from build123d import *

# Parameters (mm, degrees)
BOSS_EXTRUDE1_DEPTH                = 40.005
F_4_40_FOR_NUT_VERTICAL_DEPTH      = 82.258355524
F_4_40_FOR_NUT_VERTICAL_DEPTH_BACK = 82.258355524
SKETCH3_R                          = 1.4732
SKETCH3_R_2                        = 7.9375
SKETCH4_R                          = 3.2639
F_1_4_20_MOUNTING_DEPTH            = 82.258355524


with BuildPart() as part:
    # Sketch2 → Boss-Extrude1 (new body)
    with BuildSketch(Plane.XY):
        with BuildLine():
            Line((0, 5.842), (0, 50.0126))
            Line((0, 50.0126), (2.9972, 50.0126))
            Line((2.9972, 50.0126), (2.9972, 6.1722))
            ThreePointArc((2.9972, 6.1722), (3.92713597, 3.92713597), (6.1722, 2.9972))
            Line((6.1722, 2.9972), (50.0126, 2.9972))
            Line((50.0126, 2.9972), (50.0126, 0))
            Line((50.0126, 0), (5.842, 0))
            ThreePointArc((5.842, 0), (1.711082184, 1.711082184), (0, 5.842))
        make_face()
    extrude(amount=BOSS_EXTRUDE1_DEPTH)

    # Sketch3 → 4-40 For Nut Vertical (cut, two sides: drawn at the far end of the back side and taken through both)
    with BuildSketch(Plane.XZ.offset(-F_4_40_FOR_NUT_VERTICAL_DEPTH_BACK)):
        with Locations(Location((19.500000116, 32.7025, 0), (0, 0, 270))):
            Circle(SKETCH3_R)
        with Locations(Location((19.500000116, 7.3025, 0), (0, 0, 270))):
            Circle(SKETCH3_R)
        with Locations(Location((19.500000116, 20.0025, 0), (0, 0, 270))):
            Circle(SKETCH3_R_2)
    extrude(amount=F_4_40_FOR_NUT_VERTICAL_DEPTH + F_4_40_FOR_NUT_VERTICAL_DEPTH_BACK, mode=Mode.SUBTRACT)

    # Sketch4 → 1/4-20 Mounting (cut, through all)
    with BuildSketch(Plane.ZY):
        with Locations((7.3025, 22.0726)):
            Circle(SKETCH4_R)
        with Locations((32.7025, 22.0726)):
            Circle(SKETCH4_R)
        with Locations((20.0025, 39.8526)):
            Circle(SKETCH4_R)
    extrude(amount=-F_1_4_20_MOUNTING_DEPTH, mode=Mode.SUBTRACT)


solid = part.part
Can you work these out from the model? Positions are in its coordinate system, mm. A direction names the side the tool comes from. Coordinates: 2 decimals unless noted, no trailing zeros. Order: outer loops, then holes, each group sorted by start corner. A loop starts at its lowest first (then second) coordinate and runs counter-clockwise, first axis right, second up. Notation, with made-up numbers: (-40, 40.5) -> (7, 40.5) arc R26 cw to (7, 59.5) -> close; hole circle Ø5 at (-2.5, 77). An arc over 180 degrees is marked (long way). Use one line per item in the form item = value.
Q1. Imagine slicing it at A-A, the plane x = 19.5. List the corners of the cut face in (y, z) for me (3 decimals), then the cut area to 3 significant figures.
From the geometry:
outline = (0, 0) -> (2.997, 0) -> (2.997, 5.829) -> (0, 5.829) -> close; (0, 8.776) -> (2.997, 8.776) -> (2.997, 12.065) -> (0, 12.065) -> close; (0, 27.94) -> (2.997, 27.94) -> (2.997, 31.229) -> (0, 31.229) -> close; (0, 34.176) -> (2.997, 34.176) -> (2.997, 40.005) -> (0, 40.005) -> close
area = 54.7 mm²
Q2. Imagine slicing it at C-C, the plane y = 42. List the corners of the cut face in (x, z) for me (1 decimal), then the cut area to 3 significant figures.
From the geometry:
outline = (0, 0) -> (3, 0) -> (3, 17.5) -> (0, 17.5) -> close; (0, 22.5) -> (3, 22.5) -> (3, 40) -> (0, 40) -> close
area = 105 mm²
Q3. Which directions (+Z, -Z, +X, -X, +Y, -Y) give clear straight access to the entire face, cutting with the end or side of a thin tool? Please do faces 4 (the face through (21.88, 1.52, 12.43)), 5 (the face through (28, 2.997, 20)).
From the geometry:
face_4 = +Y, -Y
face_5 = +Z, -Z, +X, +Y
Q4. Imagine slicing it at B-B, the plane z = 22. List the corners of the cut face in (x, y) for me (3 decimals).
From the geometry:
outline = (0, 5.842) arc R5.842 ccw to (5.842, 0) -> (11.818, 0) -> (11.818, 2.997) -> (6.172, 2.997) arc R3.175 cw to (2.997, 6.172) -> (2.997, 37.271) -> (0, 37.271) -> close; (0, 42.434) -> (2.997, 42.434) -> (2.997, 50.013) -> (0, 50.013) -> close; (27.182, 0) -> (50.013, 0) -> (50.013, 2.997) -> (27.182, 2.997) -> close
Q5. We'd pull the mould along Y, two halves only. Please class faces 1 (the face through (2.997, 28, 20)), 2 (the face through (1, 50.013, 20)), 3 (the face through (1.48, 24.28, 30.3)): released by +Y, released by -Y, zero draft, split by the parting line, or undercut.
From the geometry:
face_1 = zero draft
face_2 = released by +Y
face_3 = undercut
Q6. Imagine slicing it at D-D, the plane x = 40.5. List the corners of the cut face in (y, z) for me (3 decimals), then the cut area to 3 significant figures.
From the geometry:
outline = (0, 0) -> (2.997, 0) -> (2.997, 40.005) -> (0, 40.005) -> close
area = 120 mm²
Q7. Will these pins go through, and if not, where does the flat tip stop? P1, Ø4.5, axis at x = 19.5, z = 32.7, coming from the +Y side; P2, Ø1.5, axis at y = 37, z = 6, coming from the +X side; P3, Ø5, axis at y = 7, z = 32, coming from the +X side.
From the geometry:
P1 = 3
P2 = 3
P3 = 3.47
Q8. I need wall thicknesses on L1, parallel to X at y = 18.5, z = 19; L2, parallel to Y at x = 4, z = 5. Which ranges of each line are inside material? Lowest first, please.
From the geometry:
L1 = 0 to 3
L2 = 0.3 to 3.86
